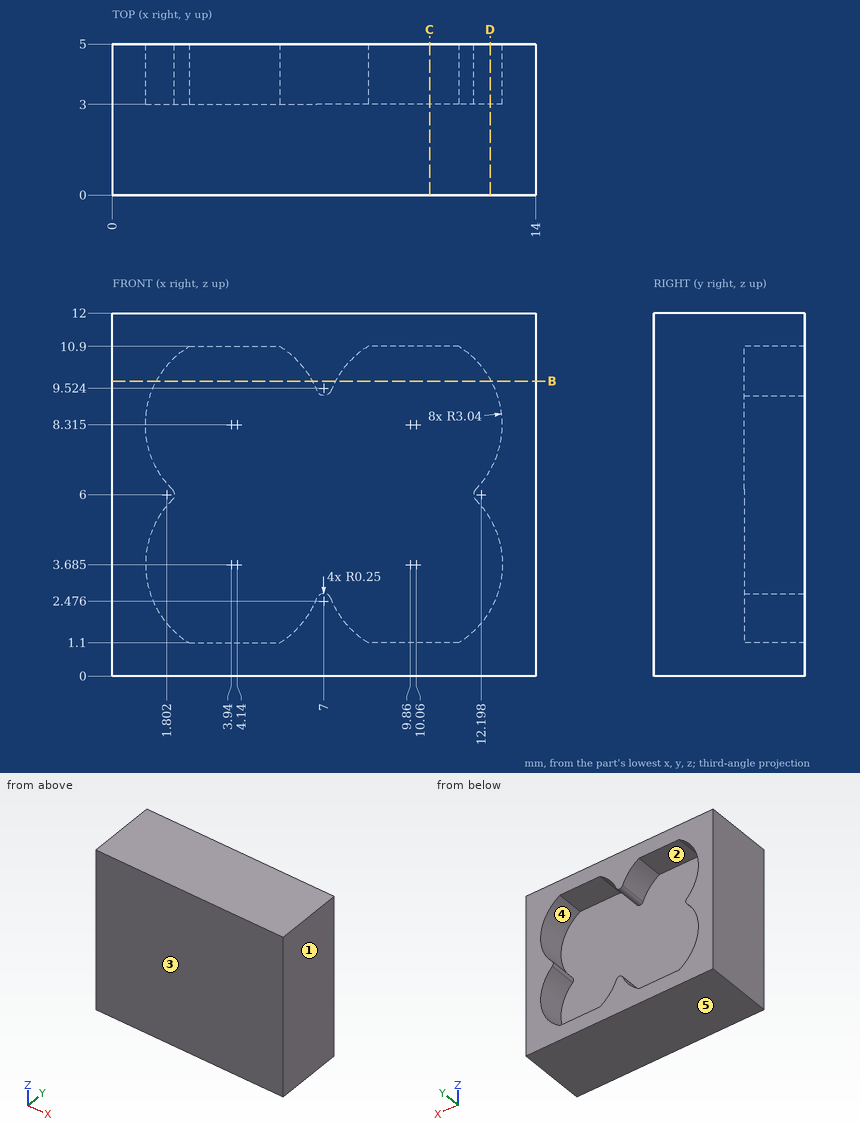
Answer from the drawing. Dimensions are ordinates in mm from the lowest x, y and z of the part. A direction names the side the tool comes from. Give positions to 0.01 mm unless a question says otherwise; leave off trailing zeros. Write each loop counter-clockwise with the first axis right and the second up, starting at its lowest first coordinate (ties: lowest second). Pieces come first, ordered by that corner, then holes. Notation, with made-up numbers: (-39.5, 89.25) - (-20.5, 89.25) arc R20 cw to (-20.5, 94.25) - close; hole circle Ø5 at (-24.5, -3). An arc over 180 degrees is marked (long way). Answer in a Markdown table with one row per item. Add a question column.
Item 1: Section B-B, the plane z = 9.75 is taken. Write down the section's boundary in (x, y).
Item 2: Find the intervals of material crossed by L1, parallel to Z at x = 8.75, y = 4.6; L2, parallel to Y at x = 5.5, z = 6; L3, parallel to X at y = 3.55, z = 3, in increasing order.
Item 3: A flat-ended cylindrical pin translates along its axis: P1, Ø5, axis at x = 9.5, z = 8, coming from the +Y side. Find the tip coordinate at first contact, or state that the pin passes through.
Item 4: A tool of negligible diameter and unlimited length cuts with its end or side. For the marked faces 1 and 2, from which of +Z, -Z, +X, -X, +Y, -Y can it reach the whole face along a straight path? Write none if from no direction.
Item 5: Determine the mould class of the marked faces 3, 4 and 5 for opening direction Z: pulls with the +Z half, pulls with the -Z half, needs draft (parallel to the pull), parting line crosses it, or undercut.
Item 6: Section D-D, the plane x = 12.5 is taken. Write down the section's boundary in (y, z).
Item 7: Section C-C, the plane x = 10.5 is taken. Write down the section's boundary in (y, z), and give its area (3 significant figures).
Recorded:
| question | item | result |
|---|---|---|
| 1 | outline | (0, 0) - (14, 0) - (14, 5) - (12.54, 5) - (12.54, 3) - (7.38, 3) - (7.38, 5) - (6.62, 5) - (6.62, 3) - (1.46, 3) - (1.46, 5) - (0, 5) - close |
| 2 | L1 | z = 0 to 1.1, 10.9 to 12 |
| 2 | L2 | y = 0 to 3 |
| 2 | L3 | x = 0 to 1.18, 12.82 to 14 |
| 3 | P1 | stops at y = 3 |
| 4 | face 1 | +Z, -Z, +X, +Y, -Y |
| 4 | face 2 | +Y |
| 5 | face 3 | needs draft |
| 5 | face 4 | undercut |
| 5 | face 5 | pulls with the -Z half |
| 6 | outline | (0, 0) - (5, 0) - (5, 2.18) - (3, 2.18) - (3, 5.19) - (5, 5.19) - (5, 6.81) - (3, 6.81) - (3, 9.82) - (5, 9.82) - (5, 12) - (0, 12) - close |
| 7 | outline | (0, 0) - (5, 0) - (5, 1.1) - (3, 1.1) - (3, 10.9) - (5, 10.9) - (5, 12) - (0, 12) - close |
| 7 | area | 40.4 mm2 |
